For this review, take the finished solid that the model builds, in its own axes (mm). Give positions to 0.01 mm unless a question says otherwise; leave off trailing zeros. Order: outer loops, then holes, each group sorted by start corner. A loop starts at its lowest first (then second) coordinate and runs counter-clockwise, first axis right, second up.
Item 1: Consider section A-A (y = 66). Give the boundary of the cut face in (x, z), plus the area to 3 significant figures.
Item 2: Consider section B-B (x = 29). Give the boundary of the cut face in (y, z), plus the area to 3 significant figures.
Item 3: For probe 1 along Y at (x, z) = (29, -0.45); probe 2 along X at (y, z) = (66.5, -0.45); probe 3 along Y at (x, z) = (2.5, -0.75), list the stretches that pass through material, from the lowest coordinate up.
Item 4: The part is to be moulded in two halves that separate along Y. For faces 1 (the flat face through (15, 31, 0)), 2 (the cylindrical face through (1.794, 65.073, -0.507)), say which applies: released by +Y, released by -Y, zero draft, split by the parting line, or undercut.
```python
from build123d import *

# Parameters (mm, degrees)
SKETCH010_W      = 4
SKETCH010_H      = 5
EXTRUDE008_DEPTH = 4
SKETCH006_W      = 35
SKETCH006_H      = 79
SKETCH006_R      = 0.95
EXTRUDE004_DEPTH = 1


with BuildPart() as led005:
    # Sketch010 → Extrude008 (new body)
    with BuildSketch(Plane(origin=(-3, 0, 0), x_dir=(0, -1, 0), z_dir=(-1, 0, 0))):
        with Locations((-5, 2.5)):
            Rectangle(SKETCH010_W, SKETCH010_H)
    extrude(amount=-EXTRUDE008_DEPTH)


with BuildPart() as cut004:
    # Sketch006 → Extrude004 (new body)
    with BuildSketch(Plane.XY.offset(-1)):
        with Locations((15.5, 30.5)):
            Rectangle(SKETCH006_W, SKETCH006_H)
        with Locations((2, -5)):
            Circle(SKETCH006_R, mode=Mode.SUBTRACT)
        with Locations((29, -5)):
            Circle(SKETCH006_R, mode=Mode.SUBTRACT)
        with Locations((2, 66)):
            Circle(SKETCH006_R, mode=Mode.SUBTRACT)
        with Locations((29, 66)):
            Circle(SKETCH006_R, mode=Mode.SUBTRACT)
    extrude(amount=EXTRUDE004_DEPTH)

    # Cut004: cut led005
    add(led005.part, mode=Mode.SUBTRACT)


solid = cut004.part
```
Resolved:
1. outline: (-2, -1) - (1.05, -1) - (1.05, 0) - (-2, 0) - close; (2.95, -1) - (28.05, -1) - (28.05, 0) - (2.95, 0) - close; (29.95, -1) - (33, -1) - (33, 0) - (29.95, 0) - close
1. area: 31.2 mm2
2. outline: (-9, -1) - (-5.95, -1) - (-5.95, 0) - (-9, 0) - close; (-4.05, -1) - (65.05, -1) - (65.05, 0) - (-4.05, 0) - close; (66.95, -1) - (70, -1) - (70, 0) - (66.95, 0) - close
2. area: 75.2 mm2
3. probe 1: y = -9 to -5.95, -4.05 to 65.05, 66.95 to 70
3. probe 2: x = -2 to 1.19, 2.81 to 28.19, 29.81 to 33
3. probe 3: y = -9 to -5.81, -4.19 to 65.19, 66.81 to 70
4. face 1: zero draft
4. face 2: undercut
